```python
from build123d import *

# Parameters (mm, degrees)
F1_DEPTH = 25.4
F2_R     = 2
F3_T     = 2


# Not quite as in the source:
# - a shell that OpenCascade refuses in one call is made with other operations: the cavity is built on its own and cut out


with BuildPart() as f1:
    # F0 (on Front) → F1 (new body)
    with BuildSketch(Plane.XZ):
        with BuildLine():
            Line((-51.5017161099, 61.5344954622), (-110.0323972047, 29.4426782099))
            ThreePointArc((-110.0323972047, 29.4426782099), (-116.6082312435, 0.741485542), (-87.3347394228, -2.4306951723))
            Line((-87.3347394228, -2.4306951723), (-45.9517985582, 35.0605621934))
            Line((-45.9517985582, 35.0605621934), (-51.5017161099, 61.5344954622))
        make_face()
    extrude(amount=F1_DEPTH)

    # F2
    f2_edges = [f1.edges().sort_by_distance(p)[0] for p in [
        (-80.767057, -25.4, 45.488587),
    ]]
    fillet(f2_edges, radius=F2_R)

    # F3: shell of thickness 2, made by hand


with BuildPart() as f3_core1:
    # F3_t2: copy of F1
    add(f1.part)

    # the walls: a layer under each face that stays
    f3_faces = [f3_core1.faces().sort_by_distance(p)[0] for p in [
        (-66.6432689905, -11.7, 16.3149335105),
        (-116.6082312435, -11.7, 0.741485542),
        (-48.7267573341, -12.7, 48.2975288278),
        (-80.7670566573, -11.7, 45.488586836),
        (-82.3442492315, -25.4, 26.9788079772),
    ]]
    thicken(f3_faces, amount=-F3_T, mode=Mode.SUBTRACT)


with BuildPart() as f1_1:
    add(f1.part)

    # what is left inside the walls is the cavity
    f3_cavity = [f3_core1.part.solids().sort_by_distance(p)[0] for p in [
        (-83.202908, -0.02, 15.807193),
    ]]
    add(f3_cavity, mode=Mode.SUBTRACT)


solid = f1_1.part
```
Geometry: final body of the model. Coordinates: model frame, mm. A direction names the side the tool comes from. Round coordinates to 2 decimals unless told otherwise and drop trailing zeros. Write each loop counter-clockwise with the first axis right and the second up, starting at its lowest first coordinate (ties: lowest second). Pieces come first, ordered by that corner, then holes. Notation, with made-up numbers: M 10.25,39 L 27.25,39 A21 ccw 27.25,50 Z; hole C 4.25,47.25 d4. An arc over 180 degrees is marked long. Answer in a Markdown table with one row per item. Add a question column.
(1) Reachability of faces 4 (the face through (-66.3, -24.8, 17.4)), 5 (the face through (-50.5, -11.5, 47)) from +Z, -Z, +X, -X, +Y, -Y: full face, straight path, thin tool, end or side. Return the list, or none.
(2) Contact query for flat-ended pins moving along their axis: pin 1 (10 mm diameter, centred on x = -107, y = -11, fed in from -Z); pin 2 (6 mm diameter, centred on y = -9, z = 49.5, fed in from +X); pin 3 (8 mm diameter, centred on x = -111.5, y = -3.5, fed in from +Z); pin 4 (8 mm diameter, centred on x = -57.5, z = 14.5, fed in from +Y). Output: stop coordinate, or through.
(3) Ray query, L1, parallel to Y at x = -72.5, z = 19.5; L2, parallel to X at y = -12.5, z = 21; L3, parallel to Z at x = -92, y = -3.25. Return the intervals inside material, ascending.
(4) Draft query along X for faces 1 (the face through (-116.87, -11.54, 1.12)), 2 (the face through (-84, -23.4, 27)), 3 (the face through (-89, 0, 40)). Return one class per face: pulls with the +X half, pulls with the -X half, needs draft (parallel to the pull), parting line crosses it, or undercut.
(5) Cut plane A-A, the plane y = -22.5. Return the cut outline in (x, z), then the cut area to 3 significant figures.
Established:
| question | item | result |
|---|---|---|
| 1 | face 4 | -Z, +X, -Y |
| 1 | face 5 | +Y |
| 2 | pin 1 | z = -7.48 |
| 2 | pin 2 | x = -48.35 |
| 2 | pin 3 | z = 30.83 |
| 2 | pin 4 | through |
| 3 | L1 | -25.4 to -23.4 |
| 3 | L2 | -118.17 to -115.9, -64.45 to -61.47 |
| 3 | L3 | -5.57 to -3.32, 37.05 to 39.33 |
| 4 | face 1 | parting line crosses it |
| 4 | face 2 | undercut |
| 4 | face 3 | needs draft |
| 5 | outline | M -110.03,29.44 A19.7 ccw long -87.33,-2.43 L -45.95,35.06 L -51.5,61.53 Z; hole M -109.07,27.69 A17.7 ccw long -88.68,-0.95 L -48.14,35.77 L -52.91,58.48 Z |
| 5 | area | 418 mm² |
